Autodesk Inventor part; units mm, degrees
ref_plane "YZ Plane" through (0, 0, 0) normal (1, 0, 0) x (0, 1, 0)
ref_plane "XZ Plane" through (0, 0, 0) normal (0, 1, 0) x (-1, 0, 0)
ref_plane "XY Plane" through (0, 0, 0) normal (0, 0, 1) x (1, 0, 0)
sketch "スケッチ1" plane through (0, 0, 0) normal (0, 0, 1) x (1, 0, 0)
  circle A0 centre (0, 0) radius 1.3
  dimension "d0" = 2.6
extrude "押し出し1" add sketch "スケッチ1" along normal blind 6
sketch "スケッチ2" plane through (0, 0, 6) normal (0, 0, 1) x (1, 0, 0)
  circle A0 centre (0, 0) radius 1.3
  circle A1 centre (0, 0) radius 2.6
  dimension "d3" = 5.2
extrude "押し出し2" add sketch "スケッチ2" along normal blind 1.5 contours A0 | A1
thread "ねじ1"
chamfer "面取り1" distance 1.3 angle 45 1 edges at (-2.6, 0, 6)
sketch "スケッチ4" plane through (0, 0, 0) normal (0, 0, -1) x (-1, 0, 0)
  circle A0 centre (0, 0) radius 1.3
extrude "押し出し4" cut sketch "スケッチ4" against normal blind 1.5
properties part number "M2.6 6mm皿ネジ" material "Steel, Mild"
Source: CAD feature listing. Evaluate the final solid. Frame: model axes, mm. A direction names the side the tool comes from. Give positions to 0.01 mm unless a question says otherwise; leave off trailing zeros. Loops run counter-clockwise (first coordinate to the right, second up) from the corner with the lowest first, then second, coordinate; pieces in that order, holes last. Notation, with made-up numbers: M 21,30.25 L 80,30.25 A29 cw 80,62.25 Z; hole C 0.5,66 d9. An arc over 180 degrees is marked long. Put each result on its own line as item: value.
Q1. Section C-C (z = 4.7). Return the cut outline in (x, y), and give its area (3 significant figures).
Response values:
outline: C 0,0 d2.6
area: 5.31 mm²
Q2. Pin query (flat end, axial travel): P1, Ø2, axis at x = 1, z = 6, coming from the +Y side; P2, Ø1, axis at y = 0, z = 6.5, coming from the -X side. Return the tip coordinate at first contact, or that it passes through.
Response values:
P1: stops at y = 2.14
P2: stops at x = -2.3
Q3. Line query: probe 1 along X at (y, z) = (-0.55, 4.25); probe 2 along Z at (x, y) = (0.1, 1.55); probe 3 along Z at (x, y) = (1.3, 0.5). Output: solid intervals per line, ascending. Write a range as [from, to].
Response values:
probe 1: x = [-1.18, 1.18]
probe 2: z = [6.25, 7.5]
probe 3: z = [6.09, 7.5]
Q4. Section D-D (z = 7). Return the cut outline in (x, y).
Response values:
outline: C 0,0 d4.6
Q5. Reachability of faces 1 (the flat face through (0, 0, 7.5)), 2 (the cylindrical face through (-0.17, -1.29, 3.72)) from +Z, -Z, +X, -X, +Y, -Y: full face, straight path, thin tool, end or side. Return the list, or none.
Response values:
face 1: +Z, +X, -X, +Y, -Y
face 2: -Z
